from build123d import *

# Parameters (mm, degrees)
MODEL_W                 = 3
MODEL_H                 = 3
SALIENTE_EXTRUIR1_DEPTH = 3


with BuildPart() as part:
    # Model → Saliente-Extruir1 (new body)
    with BuildSketch(Plane.XY):
        with BuildLine():
            Line((11.412749203, 297.239922936), (47.412749203, 297.239922936))
            ThreePointArc((47.412749203, 297.239922936), (51.912749203, 292.739922936), (47.412749203, 288.239922936))
            Line((47.412749203, 288.239922936), (11.412749203, 288.239922936))
            ThreePointArc((11.412749203, 288.239922936), (6.912749203, 292.739922936), (11.412749203, 297.239922936))
        make_face()
        with Locations((11.412749203, 292.739922936)):
            Rectangle(MODEL_W, MODEL_H, mode=Mode.SUBTRACT)
        with Locations((20.412749203, 292.739922936)):
            Rectangle(MODEL_W, MODEL_H, mode=Mode.SUBTRACT)
        with Locations((29.412749203, 292.739922936)):
            Rectangle(MODEL_W, MODEL_H, mode=Mode.SUBTRACT)
        with Locations((38.412749203, 292.739922936)):
            Rectangle(MODEL_W, MODEL_H, mode=Mode.SUBTRACT)
        with Locations((47.412749203, 292.739922936)):
            Rectangle(MODEL_W, MODEL_H, mode=Mode.SUBTRACT)
    extrude(amount=SALIENTE_EXTRUIR1_DEPTH)


solid = part.part
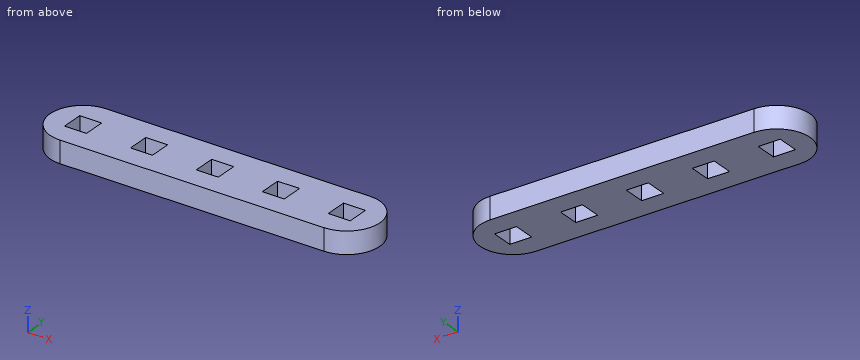
CAD build for the part. Positions are in the model's coordinates, mm. Round coordinates to 2 decimals unless told otherwise and drop trailing zeros. Write each loop counter-clockwise with the first axis right and the second up, starting at its lowest first coordinate (ties: lowest second). Pieces come first, ordered by that corner, then holes. Notation, with made-up numbers: (47.5, 34) -> (100.5, 34) arc R26 ccw to (100.5, 73) -> close; hole circle Ø1 at (53.25, 42). An arc over 180 degrees is marked (long way). Answer as a JSON object with one key per item and string values.
(1) Band-saw the part on D-D, the plane x = 48. List the corners of the cut face in (y, z).
Reported:
{"outline": "(288.28, 0) -> (291.24, 0) -> (291.24, 3) -> (288.28, 3) -> close; (294.24, 0) -> (297.2, 0) -> (297.2, 3) -> (294.24, 3) -> close"}
(2) Probe probe 1 along X at (y, z) = (292.25, 1.7); probe 2 along Y at (x, z) = (47, 0.5); probe 3 along X at (y, z) = (291.5, 2.4). List the from-to ranges inside material, lowest first. Write a range as [from, to].
Reported:
{"probe 1": "x = [6.94, 9.91], [12.91, 18.91], [21.91, 27.91], [30.91, 36.91], [39.91, 45.91], [48.91, 51.89]", "probe 2": "y = [288.24, 291.24], [294.24, 297.24]", "probe 3": "x = [7.09, 9.91], [12.91, 18.91], [21.91, 27.91], [30.91, 36.91], [39.91, 45.91], [48.91, 51.74]"}
(3) Band-saw the part on C-C, the plane y = 293.25. List the corners of the cut face in (x, z).
Reported:
{"outline": "(6.94, 0) -> (9.91, 0) -> (9.91, 3) -> (6.94, 3) -> close; (12.91, 0) -> (18.91, 0) -> (18.91, 3) -> (12.91, 3) -> close; (21.91, 0) -> (27.91, 0) -> (27.91, 3) -> (21.91, 3) -> close; (30.91, 0) -> (36.91, 0) -> (36.91, 3) -> (30.91, 3) -> close; (39.91, 0) -> (45.91, 0) -> (45.91, 3) -> (39.91, 3) -> close; (48.91, 0) -> (51.88, 0) -> (51.88, 3) -> (48.91, 3) -> close"}
(4) Band-saw the part on A-A, the plane x = 21.5. List the corners of the cut face in (y, z), then the cut area to 3 significant figures.
Reported:
{"outline": "(288.24, 0) -> (291.24, 0) -> (291.24, 3) -> (288.24, 3) -> close; (294.24, 0) -> (297.24, 0) -> (297.24, 3) -> (294.24, 3) -> close", "area": "18.0 mm^2"}
(5) Band-saw the part on B-B, the plane z = 0.7. List the corners of the cut face in (x, y).
Reported:
{"outline": "(11.41, 288.24) -> (47.41, 288.24) arc R4.5 ccw to (47.41, 297.24) -> (11.41, 297.24) arc R4.5 ccw to start; hole (9.91, 291.24) -> (12.91, 291.24) -> (12.91, 294.24) -> (9.91, 294.24) -> close; hole (18.91, 291.24) -> (21.91, 291.24) -> (21.91, 294.24) -> (18.91, 294.24) -> close; hole (27.91, 291.24) -> (30.91, 291.24) -> (30.91, 294.24) -> (27.91, 294.24) -> close; hole (36.91, 291.24) -> (39.91, 291.24) -> (39.91, 294.24) -> (36.91, 294.24) -> close; hole (45.91, 291.24) -> (48.91, 291.24) -> (48.91, 294.24) -> (45.91, 294.24) -> close"}
(6) Pin check, flat tip, straight feed: P1, Ø1.5, axis at y = 292.5, z = 1.5, coming from the -X side. Stop position of the tip, or through.
Reported:
{"P1": "stops at x = 6.91"}
